```python
from build123d import *

# Parameters (mm, degrees)
F0_R            = 11.175
F1_DEPTH        = 7
F2_COUNT        = 3
F4_DEPTH        = 7
F4_COPIES_COUNT = 3
F5_SIZE         = 2
F6_SIZE         = 2
F7_SIZE         = 2


# Not quite as in the source:
# - a pattern or mirror of a feature is missing from the dataset's text; its kind, count and spacing are read off the source's solid


with BuildPart() as f1:
    # F0 (on Top) → F1 (new body)
    with BuildSketch(Plane.XY):
        with BuildLine():
            ThreePointArc((-8.3372222223, 8.8987877603), (-4.8493412747, -11.1884577663), (12.1941665556, 0))
            ThreePointArc((12.1941665556, 0), (11.1884577663, 4.8493412747), (8.3372222223, 8.8987877603))
            ThreePointArc((8.3372222223, 8.8987877603), (0, 12.1941665556), (-8.3372222223, 8.8987877603))
        make_face()
        Circle(F0_R, mode=Mode.SUBTRACT)
        with BuildLine():
            ThreePointArc((-8.3372222223, 8.8987877603), (0, 12.1941665556), (8.3372222223, 8.8987877603))
            Line((8.3372222223, 8.8987877603), (20.9652856439, 34.0654780954))
            ThreePointArc((20.9652856439, 34.0654780954), (0, 40.0055861953), (-20.9652856439, 34.0654780954))
            Line((-20.9652856439, 34.0654780954), (-8.3372222223, 8.8987877603))
        make_face()
        with Locations((0, 25.5817994475)):
            Circle(F0_R, mode=Mode.SUBTRACT)
    extrude(amount=F1_DEPTH)

    # F2: F1 ×3 about axis
    f2_axis = Axis((0, 0, 0), (0, 0, -1))


with BuildPart() as f1_1:
    add(f1.part)
    for i in range(1, F2_COUNT):
        add(f1.part.rotate(f2_axis, i * 360 / F2_COUNT))

    # F3 (on face) → F4 (join)
    with BuildSketch(Plane.XY.offset(7)):
        with BuildLine():
            Line((-8.5294263987, -19.2529557346), (-9.9039361375, -21.3411901509))
            ThreePointArc((-9.9039361375, -21.3411901509), (0, -24.0747086913), (9.9039361375, -21.3411901509))
            Line((9.9039361375, -21.3411901509), (8.5294263987, -19.2529557346))
            ThreePointArc((8.5294263987, -19.2529557346), (0, -21.1847607817), (-8.5294263987, -19.2529557346))
        make_face()
    f4 = extrude(amount=-F4_DEPTH)

    # F4_copies: F4 ×3 about axis
    f4_copies_axis = Axis((0, 0, 0), (0, 0, 1))
    for i in range(1, F4_COPIES_COUNT):
        add(f4.rotate(f4_copies_axis, i * 360 / F4_COPIES_COUNT))

    # F5
    f5_edges = [f1_1.edges().sort_by_distance(p)[0] for p in [
        (34.645854, -20.002793, 7),
        (34.645854, -20.002793, 0),
    ]]
    chamfer(f5_edges, length=F5_SIZE)

    # F6
    f6_edges = [f1_1.edges().sort_by_distance(p)[0] for p in [
        (-34.645854, -20.002793, 7),
        (-34.645854, -20.002793, 0),
    ]]
    chamfer(f6_edges, length=F6_SIZE)

    # F7
    f7_edges = [f1_1.edges().sort_by_distance(p)[0] for p in [
        (0, 40.005586, 7),
        (0, 40.005586, 0),
    ]]
    chamfer(f7_edges, length=F7_SIZE)


solid = f1_1.part
```
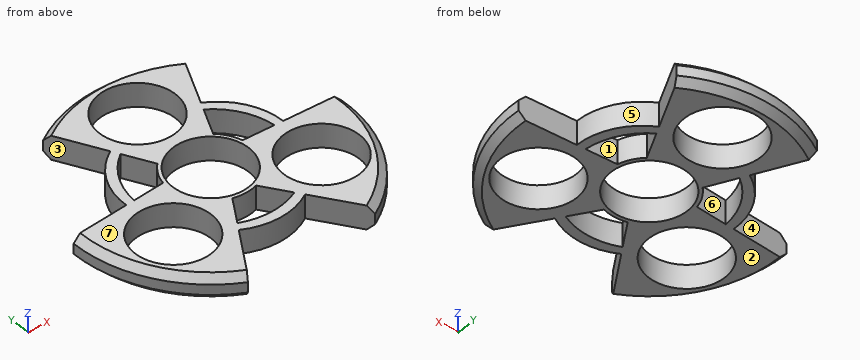
Geometry: final body of the model. Coordinates: model frame, mm. Face numbers are marked on the shaded views. A direction names the side the tool comes from. Round coordinates to 2 decimals unless told otherwise and drop trailing zeros. Order: outer loops, then holes, each group sorted by start corner. A loop starts at its lowest first (then second) coordinate and runs counter-clockwise, first axis right, second up. Notation, with made-up numbers: (76.25, -26.75) -> (108.25, -26.75) arc R31 cw to (108.25, -1.75) -> close; hole circle Ø5 at (-26.75, -4.75). An arc over 180 degrees is marked (long way). Use one line per item in the form item = value.
(1) Draft query along X for the marked faces 4, 5, 6 and 7. Return one class per face: pulls with the +X half, pulls with the -X half, needs draft (parallel to the pull), parting line crosses it, or undercut.
Results list:
face_4 = pulls with the -X half
face_5 = pulls with the +X half
face_6 = undercut
face_7 = needs draft
(2) Section A-A on x = 0. Return loops of the section in (y, z) (3 decimals), and give its area (3 significant figures).
Results list:
outline = (-24.075, 0) -> (-21.185, 0) -> (-21.185, 7) -> (-24.075, 7) -> close; (-12.194, 0) -> (-11.175, 0) -> (-11.175, 7) -> (-12.194, 7) -> close; (11.175, 0) -> (14.407, 0) -> (14.407, 7) -> (11.175, 7) -> close; (36.757, 0) -> (38.006, 0) -> (40.006, 2) -> (40.006, 5) -> (38.006, 7) -> (36.757, 7) -> close
area = 68.7 mm^2
(3) Section C-C on z = 3. Return loops of the section in (x, y) (3 decimals).
Results list:
outline = (-39.984, 1.124) arc R39.968 ccw to (-19.019, -35.189) -> (-9.904, -21.341) arc R19.308 ccw to (9.904, -21.341) -> (19.019, -35.189) arc R39.968 ccw to (39.984, 1.124) -> (23.434, 2.094) arc R19.308 ccw to (13.53, 19.248) -> (20.965, 34.065) arc R39.968 ccw to (-20.965, 34.065) -> (-13.53, 19.248) arc R19.308 ccw to (-23.434, 2.094) -> close; hole circle Ø22.35 at (-22.154, -12.791); hole (-20.938, 2.24) -> (-11.875, 2.771) arc R12.194 cw to (-8.337, 8.899) -> (-12.409, 17.013) arc R19.796 ccw to start; hole circle Ø22.35 at (0, 0); hole circle Ø22.35 at (0, 25.582); hole (-8.529, -19.253) arc R19.796 ccw to (8.529, -19.253) -> (3.538, -11.67) arc R12.194 cw to (-3.538, -11.67) -> close; hole (8.337, 8.899) arc R12.194 cw to (11.875, 2.771) -> (20.938, 2.24) arc R19.796 ccw to (12.409, 17.013) -> close; hole circle Ø22.35 at (22.154, -12.791)
(4) Section D-D on y = 15.5. Return loops of the section in (x, z), and give its area (3 significant figures).
Results list:
outline = (-18.3, 0) -> (-14.34, 0) -> (-14.34, 7) -> (-18.3, 7) -> close; (-11.65, 0) -> (-4.82, 0) -> (-4.82, 7) -> (-11.65, 7) -> close; (4.82, 0) -> (11.65, 0) -> (11.65, 7) -> (4.82, 7) -> close; (14.34, 0) -> (18.3, 0) -> (18.3, 7) -> (14.34, 7) -> close
area = 151 mm^2
(5) Access query for the marked faces 1, 2 and 3. Directions: +Z, -Z, +X, -X, +Y, -Y. A direction counts if a zero-diameter tool reaches every point of the face in a straight line with its end or side. Return the directions, or none.
Results list:
face_1 = +Z, -Z
face_2 = -Z, +X, -X, +Y, -Y
face_3 = +Z, -Z, -X
(6) Section B-B on y = 7. Return loops of the section in (x, z), and give its area (3 significant figures).
Results list:
outline = (-22.88, 0) -> (-19.97, 0) -> (-19.97, 7) -> (-22.88, 7) -> close; (-9.98, 0) -> (-8.71, 0) -> (-8.71, 7) -> (-9.98, 7) -> close; (8.71, 0) -> (9.98, 0) -> (9.98, 7) -> (8.71, 7) -> close; (19.97, 0) -> (22.88, 0) -> (22.88, 7) -> (19.97, 7) -> close
area = 58.6 mm^2
(7) First-contact query: pin 1 Ø13.5 at (x, y) = (0, 0) entering from +Z. Flat tip, straight axial feed; report the tip coordinate or a pass-through.
Results list:
pin_1 = through
(8) Ray query, probe 1 along X at (y, z) = (0, 2) (3 decimals); probe 2 along X at (y, z) = (-14, 2); probe 3 along X at (y, z) = (4, 0.75). Return the intervals inside material, ascending. Write a range as [from, to].
Results list:
probe_1 = [-40.001, -11.175], [11.175, 40.001]
probe_2 = [-37.48, -33.26], [-11.05, -5.07], [5.07, 11.05], [33.26, 37.48]
probe_3 = [-23.37, -20.72], [-11.52, -10.43], [10.43, 11.52], [20.72, 23.37]
